Could you check a few things on this model? Use its own coordinates, in mm. A direction names the side the tool comes from. Give positions to 0.01 mm unless a question says otherwise; leave off trailing zeros. Loops run counter-clockwise (first coordinate to the right, second up) from the corner with the lowest first, then second, coordinate; pieces in that order, holes last. Notation, with made-up numbers: M 38.5,34 L 80.5,34 A15 ccw 80.5,40 Z; hole C -19,43 d1. An arc over 180 degrees is marked long. Answer in a Markdown table with one row per item. Add a question column.
1. Which directions (+Z, -Z, +X, -X, +Y, -Y) give clear straight access to the entire face, cutting with the end or side of a thin tool? Please do faces 1 (the flat face through (89.902, -52, 8)), 2 (the flat face through (-87.098, -58, 9)), 3 (the flat face through (95.8, -59.673, -0.6)), 4 (the flat face through (-89.098, -50, 8)), 5 (the flat face through (-89, -50, 16)).
2. I'm going to push flat-ended pins straight in: pin 1 Ø1.7 at (x, y) = (-137.1, -45.67) entering from +Z; pin 2 Ø3 at (x, y) = (91, 40.5) entering from -Z; pin 3 Ø1.5 at (y, z) = (88.5, 0.5) entering from -X; pin 4 Ø1 at (y, z) = (-42, 7) entering from +X. Where does each tip first touch, or does it pass through?
3. I need wall thicknesses on line 1 along Z through (x, y) = (-101.5, 36). Which ranges of the line are inside material? Lowest first, please. Write a range as from..to.
4. If we section it at B-B on y = -31.5: List the corners of the cut face in (x, z) for me.
5. If we section it at C-C on x = -67: List the corners of the cut face in (y, z) for me, then the cut area to 3 significant figures.
6. If we section it at A-A on z = 8.5: List the corners of the cut face in (x, y) for me, then the cut area to 3 significant figures.
7. Thinking about a two-plate mould opening in X: for faces 6 (the flat face through (-91.098, -52, 8)), 7 (the flat face through (-3, 30, -1)), 8 (the flat face through (85.902, -58, 9)), 9 (the flat face through (-27.2, -42.673, -0.6)), which applies, released by +X, released by -X, zero draft, split by the parting line, or undercut?
```python
from build123d import *

# Parameters (mm, degrees)
F2_DEPTH = 16
F4_DEPTH = 1
F5_W     = 2
F5_H     = 2
F6_DEPTH = 20
F7_W     = 2
F7_H     = 12
F8_DEPTH = 2
F10_D    = 1.5
F11_R    = 3


with BuildPart() as f2:
    # F1 (on Top) → F2 (new body)
    with BuildSketch(Plane.XY):
        Polygon((-91.098284, -40.672917), (-91.098284, -59.672917), (-89.098284, -59.672917), (-89.098284, -45.672917), (-86.098284, -45.672917), (-86.098284, -43.672917), (-89.098284, -43.672917), (-89.098284, -42.672917), (-86.098284, -42.672917), (-86.098284, -40.672917), align=None)
        Polygon((84.901716, -42.672917), (87.901716, -42.672917), (87.901716, -43.672917), (84.901716, -43.672917), (84.901716, -45.672917), (87.901716, -45.672917), (87.901716, -59.672917), (89.901716, -59.672917), (89.901716, -40.672917), (84.901716, -40.672917), align=None)
    extrude(amount=F2_DEPTH)

    # F3 (on Top) → F4 (join)
    with BuildSketch(Plane.XY):
        Polygon((-139.098284, -59.672917), (-89.098284, -59.672917), (-89.098284, -42.672917), (87.901716, -42.672917), (87.901716, -59.672917), (137.901716, -59.672917), (137.901716, 117.327083), (-139.098284, 117.327083), align=None)
    extrude(amount=-F4_DEPTH)

    # F5 (on face) → F6 (join)
    with BuildSketch(Plane.XY.offset(16)):
        with Locations((-88.098284, -58.672917)):
            Rectangle(F5_W, F5_H)
        with Locations((86.901716, -58.672917)):
            Rectangle(F5_W, F5_H)
    extrude(amount=-F6_DEPTH)

    # F7 (on face) → F8 (join)
    with BuildSketch(Plane.XY.offset(16)):
        with Locations((-88.098284, -51.672917)):
            Rectangle(F7_W, F7_H)
        with Locations((86.901716, -51.672917)):
            Rectangle(F7_W, F7_H)
    extrude(amount=-F8_DEPTH)

    # F10 (through all)
    with Locations(Plane.XY):
        with Locations((-49.598284, 115.327083), (-137.098284, 31.327083), (-137.098284, -57.172917), (-137.098284, -45.672917), (-137.098284, 115.327083), (135.901716, -45.672917), (-96.098284, -57.172917), (94.901716, -57.172917), (135.901716, -57.172917), (48.401716, 115.327083), (135.901716, 115.327083), (135.901716, 31.327083)):
            Hole(F10_D / 2)

    # F11
    f11_edges = [f2.edges().sort_by_distance(p)[0] for p in [
        (-139.098284, 117.327083, -0.5),
        (137.901716, 117.327083, -0.5),
        (-91.098284, -40.672917, 8),
        (-139.098284, -59.672917, -0.5),
        (89.901716, -40.672917, 8),
        (137.901716, -59.672917, -0.5),
    ]]
    fillet(f11_edges, radius=F11_R)


solid = f2.part
```
Results:
| question | item | result |
|---|---|---|
| 1 | face 1 | +Z, +X, +Y, -Y |
| 1 | face 2 | +Z, -Z, -Y |
| 1 | face 3 | +Z, -Z, +X, -X, -Y |
| 1 | face 4 | -Z |
| 1 | face 5 | +Z, +X, -X, +Y, -Y |
| 2 | pin 1 | z = 0 |
| 2 | pin 2 | z = -1 |
| 2 | pin 3 | x = -139.1 |
| 2 | pin 4 | x = 89.66 |
| 3 | line 1 | -1..0 |
| 4 | outline | M -139.1,-1 L 137.9,-1 L 137.9,0 L -139.1,0 Z |
| 5 | outline | M -42.67,-1 L 117.33,-1 L 117.33,0 L -42.67,0 Z |
| 5 | area | 160 mm2 |
| 6 | outline | M -91.1,-59.67 L -87.1,-59.67 L -87.1,-57.67 L -89.1,-57.67 L -89.1,-45.67 L -86.1,-45.67 L -86.1,-43.67 L -89.1,-43.67 L -89.1,-42.67 L -86.1,-42.67 L -86.1,-40.67 L -88.1,-40.67 A3 ccw -91.1,-43.67 Z; M 84.9,-45.67 L 87.9,-45.67 L 87.9,-57.67 L 85.9,-57.67 L 85.9,-59.67 L 89.9,-59.67 L 89.9,-43.67 A3 ccw 86.9,-40.67 L 84.9,-40.67 L 84.9,-42.67 L 87.9,-42.67 L 87.9,-43.67 L 84.9,-43.67 Z |
| 6 | area | 104 mm2 |
| 7 | face 6 | released by -X |
| 7 | face 7 | zero draft |
| 7 | face 8 | undercut |
| 7 | face 9 | undercut |
